Source: CAD feature listing. Evaluate the final solid. Frame: model axes, mm. Give positions to 0.01 mm unless a question says otherwise; leave off trailing zeros. Loops run counter-clockwise (first coordinate to the right, second up) from the corner with the lowest first, then second, coordinate; pieces in that order, holes last.
```python
from build123d import *

# Parameters (mm, degrees)
MAIN_PROFILE_SKETCH_W = 6
MAIN_PROFILE_SKETCH_H = 7.25
MAIN_PROFILE_SKETCH_R = 1.1
MAIN_EXTRUSION_DEPTH  = 1


with BuildPart() as part:
    # Main Profile Sketch → Main Extrusion (new body)
    with BuildSketch(Plane(origin=(0, -203.2, 0), x_dir=(-1, 0, 0), z_dir=(0, -1, 0))):
        with Locations((19.009182883, 67.119882879)):
            Rectangle(MAIN_PROFILE_SKETCH_W, MAIN_PROFILE_SKETCH_H)
        with Locations(Location((19.009182883, 67.744882879, 0), (0, 0, 90))):
            Circle(MAIN_PROFILE_SKETCH_R, mode=Mode.SUBTRACT)
    extrude(amount=MAIN_EXTRUSION_DEPTH)


solid = part.part
```
(1) Section B-B, the plane z = -67. Return the cut outline in (x, y).
A:
outline: (-22.01, -204.2) - (-19.82, -204.2) - (-19.82, -203.2) - (-22.01, -203.2) - close; (-18.2, -204.2) - (-16.01, -204.2) - (-16.01, -203.2) - (-18.2, -203.2) - close
(2) Mould query, pull axis Z, two halves, no side actions, for faces 1 (the cylindrical face through (-19.43, -203.69, -68.76)), 2 (the flat face through (-19, -204, -70.745)), 3 (the flat face through (-16.009, -204, -67)). Classes: pulls with the +Z half, pulls with the -Z half, needs draft (parallel to the pull), parting line crosses it, or undercut.
A:
face 1: undercut
face 2: pulls with the -Z half
face 3: needs draft
(3) Ray query, line 1 along X through (y, z) = (-203.35, -68); line 2 along Z through (x, y) = (-18.8, -203.9); line 3 along Z through (x, y) = (-19.7, -204). Return the intervals inside material, ascending.
A:
line 1: x = -22.01 to -20.08, -17.94 to -16.01
line 2: z = -70.74 to -68.82, -66.66 to -63.49
line 3: z = -70.74 to -68.6, -66.89 to -63.49
(4) Section A-A, the plane x = -18.7. Return the cut outline in (y, z).
A:
outline: (-204.2, -70.74) - (-203.2, -70.74) - (-203.2, -68.8) - (-204.2, -68.8) - close; (-204.2, -66.69) - (-203.2, -66.69) - (-203.2, -63.49) - (-204.2, -63.49) - close
(5) Section C-C, the plane y = -203.35. Return the cut outline in (x, z), then the cut area to 3 significant figures.
A:
outline: (-22.01, -70.74) - (-16.01, -70.74) - (-16.01, -63.49) - (-22.01, -63.49) - close; hole circle Ø2.2 at (-19.01, -67.74)
area: 39.7 mm2
